Design review of the part shown in the three views and the two pictorial views. Dimensions are in mm from the part's minimum x, y and z. A direction names the side the tool comes from. Coordinates: 2 decimals unless noted, no trailing zeros. Loops run counter-clockwise (first coordinate to the right, second up) from the corner with the lowest first, then second, coordinate; pieces in that order, holes last. Notation, with made-up numbers: (79.25, 52) -> (90.25, 52) arc R31 ccw to (90.25, 77) -> close; hole circle Ø10 at (-37.75, -10.75). An arc over 180 degrees is marked (long way). Use a Markdown table: item, result. Add a question column.
Q1. Take a section at C-C on x = 63. Write out the cut boundary in (y, z).
Q2. Draft analysis for pull direction Z (two halves, no side actions). For the marked faces 1, 2 and 3, state which applies: pulls with the +Z half, pulls with the -Z half, needs draft (parallel to the pull), parting line crosses it, or undercut.
Q3. Take a section at B-B on z = 50. Write out the cut boundary in (x, y).
Q4. For the marked faces 4, 5 and 6, list the 3-axis set-ups (+Z, -Z, +X, -X, +Y, -Y) from which the entire face can be reached by the end or side of a thin tool; tool diameter is ignored.
Q5. Clearance check with flat-ended pins moving along their axes: pin 1 Ø6 at (y, z) = (24, 41.5) entering from +X; pin 2 Ø1.2 at (x, y) = (73, 16.5) entering from -Z; pin 3 Ø10 at (y, z) = (5, 47.5) entering from -X; pin 4 Ø8 at (x, z) = (86.5, 71) entering from -Y. State where each tip first meets the part, or that it passes through.
Q6. Take a section at D-D on y = 26. Write out the cut boundary in (x, z).
Q7. For probe 1 along Z at (x, y) = (34.5, 11.5); probe 2 along X at (y, z) = (9.5, 42.5); probe 3 along Y at (x, z) = (54.5, 58.5), list the stretches that pass through material, from the lowest coordinate up.
Q8. Take a section at A-A on y = 19.5. Write out the cut boundary in (x, z), plus the area to 3 significant figures.
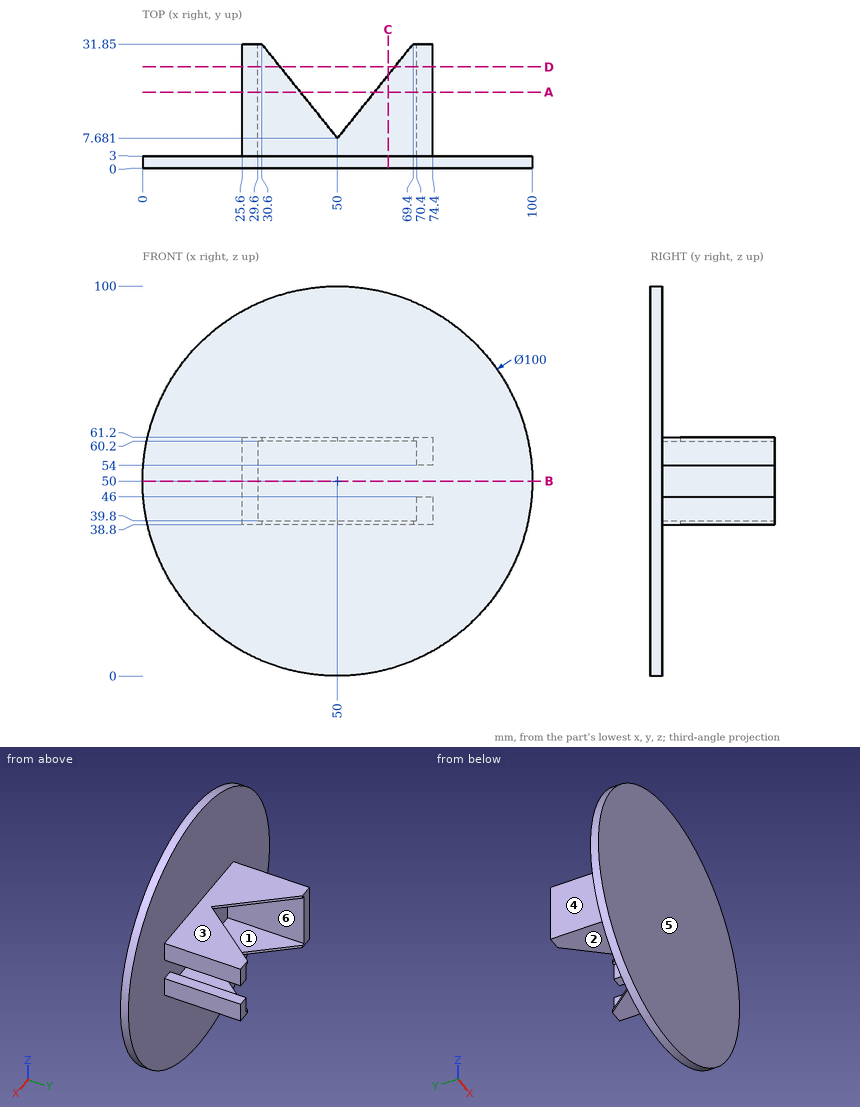
Answer list:
| question | item | result |
|---|---|---|
| 1 | outline | (0, 1.72) -> (3, 1.72) -> (3, 38.8) -> (23.88, 38.8) -> (23.88, 39.8) -> (3, 39.8) -> (3, 60.2) -> (23.88, 60.2) -> (23.88, 61.2) -> (3, 61.2) -> (3, 98.28) -> (0, 98.28) -> close |
| 2 | face 1 | undercut |
| 2 | face 2 | pulls with the -Z half |
| 2 | face 3 | pulls with the +Z half |
| 3 | outline | (0, 0) -> (100, 0) -> (100, 3) -> (29.6, 3) -> (29.6, 31.85) -> (25.6, 31.85) -> (25.6, 3) -> (0, 3) -> close |
| 4 | face 4 | +Z, -Z, -X, +Y |
| 4 | face 5 | +Z, -Z, +X, -X, -Y |
| 4 | face 6 | +Y |
| 5 | pin 1 | x = 74.4 |
| 5 | pin 2 | z = 38.8 |
| 5 | pin 3 | x = 0 |
| 5 | pin 4 | y = 0 |
| 6 | outline | (25.6, 38.8) -> (35.3, 38.8) -> (35.3, 39.8) -> (29.6, 39.8) -> (29.6, 60.2) -> (35.3, 60.2) -> (35.3, 61.2) -> (25.6, 61.2) -> close; (64.7, 38.8) -> (74.4, 38.8) -> (74.4, 46) -> (70.4, 46) -> (70.4, 39.8) -> (64.7, 39.8) -> close; (64.7, 60.2) -> (70.4, 60.2) -> (70.4, 54) -> (74.4, 54) -> (74.4, 61.2) -> (64.7, 61.2) -> close |
| 7 | probe 1 | 38.8 to 39.8, 60.2 to 61.2 |
| 7 | probe 2 | 25.6 to 29.6, 70.4 to 74.4 |
| 7 | probe 3 | 0 to 3 |
| 8 | outline | (25.6, 38.8) -> (40.51, 38.8) -> (40.51, 39.8) -> (29.6, 39.8) -> (29.6, 60.2) -> (40.51, 60.2) -> (40.51, 61.2) -> (25.6, 61.2) -> close; (59.49, 38.8) -> (74.4, 38.8) -> (74.4, 46) -> (70.4, 46) -> (70.4, 39.8) -> (59.49, 39.8) -> close; (59.49, 60.2) -> (70.4, 60.2) -> (70.4, 54) -> (74.4, 54) -> (74.4, 61.2) -> (59.49, 61.2) -> close |
| 8 | area | 191 mm² |
